```python
from build123d import *

# Parameters (mm, degrees)
SKETCH1_R           = 12.7
BOSS_EXTRUDE1_DEPTH = 47
SKETCH2_W           = 14
SKETCH2_H           = 2
BOSS_EXTRUDE2_DEPTH = 6.2
SKETCH3_W           = 14
SKETCH3_H           = 1.6
CUT_EXTRUDE1_DEPTH  = 6.2


with BuildPart() as part:
    # Sketch1 → Boss-Extrude1 (new body)
    with BuildSketch(Plane.XY):
        Circle(SKETCH1_R)
    extrude(amount=BOSS_EXTRUDE1_DEPTH)

    # Sketch2 → Boss-Extrude2 (add)
    with BuildSketch(Plane(origin=(0, 0, 0), x_dir=(-1, 0, 0), z_dir=(0, 0, -1))):
        Rectangle(SKETCH2_W, SKETCH2_H)
    extrude(amount=BOSS_EXTRUDE2_DEPTH)

    # Sketch3 → Cut-Extrude1 (cut)
    with BuildSketch(Plane(origin=(0, 0, -6.2), x_dir=(-1, 0, 0), z_dir=(0, 0, -1))):
        Rectangle(SKETCH3_W, SKETCH3_H)
    extrude(amount=-CUT_EXTRUDE1_DEPTH, mode=Mode.SUBTRACT)


solid = part.part
```
Part model, mm, in its own coordinate system. A direction names the side the tool comes from. Round coordinates to 2 decimals unless told otherwise and drop trailing zeros. Order: outer loops, then holes, each group sorted by start corner. A loop starts at its lowest first (then second) coordinate and runs counter-clockwise, first axis right, second up. Notation, with made-up numbers: M -11.75,72.5 L 10.25,72.5 A12 cw 10.25,77.5 Z; hole C 13,-21.75 d1. An arc over 180 degrees is marked long. Put each result on its own line as item: value. Start each with the question number.
1. Tool access for faces 4 (the face through (-2.75, -12.4, 23.17)), 5 (the face through (0, -0.8, -3)), 6 (the face through (0, -1, -3)): list every direction of +Z, -Z, +X, -X, +Y, -Y with a clear straight run to the whole face (end or side of a thin tool).
2. Slice it at C-C on z = 36. List the corners of the cut face in (x, y), then the cut area to 3 significant figures.
3. Slice it at D-D on x = 4.5. List the corners of the cut face in (y, z).
4. Drill centre lines: probe 1 along Z at (x, y) = (-8.25, 7); probe 2 along Y at (x, z) = (0, 18.5); probe 3 along Y at (x, z) = (-4, 35). Where is each one in solid material? Low to high. Write a range as [from, to].
5. Slice it at B-B on y = 0. List the corners of the cut face in (x, z).
6. Slice it at A-A on x = 0. List the corners of the cut face in (y, z), then the cut area to 3 significant figures.
7. Two-plate mould, pull along Y, no slides. Class faces 1 (the face through (0, 0, 47)), 2 (the face through (0, 0.8, -3)), 3 (the face through (0, 1, -3)): +Y half, -Y half, draft (parallel to the pull), parting line (faces both ways), or undercut.
8. Drop flat-ended pins along their axis: pin 1 (3 mm diameter, centred on x = 0, z = -2, fed in from -Y); pin 2 (6 mm diameter, centred on y = -6, z = 4.5, fed in from -X); pin 3 (5 mm diameter, centred on y = 8, z = 22.5, fed in from -X). Give the stop position or say it passes through.
Findings:
1. face 4: +Z, -Z
1. face 5: -Z, +X, -X
1. face 6: -Z, +X, -X, -Y
2. outline: C 0,0 d25.4
2. area: 507 mm2
3. outline: M -11.88,0 L -1,0 L -1,-6.2 L -0.8,-6.2 L -0.8,0 L 0.8,0 L 0.8,-6.2 L 1,-6.2 L 1,0 L 11.88,0 L 11.88,47 L -11.88,47 Z
4. probe 1: [0, 47]
4. probe 2: [-12.7, 12.7]
4. probe 3: [-12.05, 12.05]
5. outline: M -12.7,0 L 12.7,0 L 12.7,47 L -12.7,47 Z
6. outline: M -12.7,0 L -1,0 L -1,-6.2 L -0.8,-6.2 L -0.8,0 L 0.8,0 L 0.8,-6.2 L 1,-6.2 L 1,0 L 12.7,0 L 12.7,47 L -12.7,47 Z
6. area: 1,200 mm2
7. face 1: draft
7. face 2: undercut
7. face 3: +Y half
8. pin 1: y = -1
8. pin 2: x = -12.34
8. pin 3: x = -11.45
